```python
from build123d import *

# Parameters (mm, degrees)
F1_W     = 127
F1_H     = 127
F2_DEPTH = 127
F3_W     = 127
F3_H     = 127
F4_DEPTH = 245.872


# Not quite as in the source:
# - a variable given as a bare number and used for a length is read in inches; the dataset says mm whatever the document's units were


with BuildPart() as f2:
    # F1 (on Front) → F2 (new body)
    with BuildSketch(Plane.XZ):
        with Locations((-59.2341877744, -35.8161340777)):
            Rectangle(F1_W, F1_H)
    extrude(amount=F2_DEPTH)

    # F3 (on face) → F4 (join)
    with BuildSketch(Plane.XZ.offset(127)):
        with Locations((-186.2341877744, -35.8161340777)):
            Rectangle(F3_W, F3_H)
    extrude(amount=-F4_DEPTH)


solid = f2.part
```
Source: CAD feature listing. Evaluate the final solid. Frame: model axes, mm. A direction names the side the tool comes from. Coordinates: 2 decimals unless noted, no trailing zeros. Loops run counter-clockwise (first coordinate to the right, second up) from the corner with the lowest first, then second, coordinate; pieces in that order, holes last. Notation, with made-up numbers: M 72.5,75 L 107.5,75 A29 ccw 107.5,98 Z; hole C -24.5,3 d4. An arc over 180 degrees is marked long. Use CSV: the item, a comma, the result in double quotes.
(1) Line query: line 1 (Y direction, x = -105.5, z = -25); line 2 (X direction, y = 5.5, z = -7). Output: solid intervals per line, ascending. Write a range as [from, to].
Answers follow:
line 1,"[-127, 0]"
line 2,"[-249.73, -122.73]"
(2) Cut plane B-B on x = -67.5. Return loops of the section in (y, z), and give its area (3 significant figures).
Answers follow:
outline,"M -127,-99.32 L 0,-99.32 L 0,27.68 L -127,27.68 Z"
area,"16,100 mm²"
(3) Cut plane A-A on z = -8. Return loops of the section in (x, y).
Answers follow:
outline,"M -249.73,-127 L 4.27,-127 L 4.27,0 L -122.73,0 L -122.73,118.87 L -249.73,118.87 Z"
(4) Cut plane C-C on y = 82. Return loops of the section in (x, z), and give its area (3 significant figures).
Answers follow:
outline,"M -249.73,-99.32 L -122.73,-99.32 L -122.73,27.68 L -249.73,27.68 Z"
area,"16,100 mm²"
(5) Reachability of faces 1 (the face through (-60, 0, -35)), 2 (the face through (-187, 118.872, -35)) from +Z, -Z, +X, -X, +Y, -Y: full face, straight path, thin tool, end or side. Return the list, or none.
Answers follow:
face 1,"+Z, -Z, +X, +Y"
face 2,"+Z, -Z, +X, -X, +Y"
